The listing builds one solid part. Answer for the finished solid, in the listing's coordinates (mm). A direction names the side the tool comes from. Round coordinates to 2 decimals unless told otherwise and drop trailing zeros. Order: outer loops, then holes, each group sorted by start corner. A loop starts at its lowest first (then second) coordinate and runs counter-clockwise, first axis right, second up. Notation, with made-up numbers: (-4, -21) - (6, -21) arc R16 ccw to (6, 7) - close; hole circle Ø6 at (28, 39.25). An arc over 180 degrees is marked (long way). Write item = value, one per line.
from build123d import *

# Parameters (mm, degrees)
SKETCH1_R           = 2.25
SKETCH1_R_2         = 6.35
BOSS_EXTRUDE1_DEPTH = 12.7
FILLET1_R           = 6.35
FILLET3_R           = 6.35
FILLET5_R           = 2.5
FILLET4_R           = 1
CUT_EXTRUDE1_REACH  = 104.568
SKETCH2_R           = 2.25


with BuildPart() as part:
    # Sketch1 → Boss-Extrude1 (new body)
    # profile 1 of 2: a face of its own
    with BuildSketch(Plane(origin=(0, 0, 0), x_dir=(0, 0, -1), z_dir=(1, 0, 0))):
        with BuildLine():
            Line((-6.35, 76.319743879), (-6.35, 11.3))
            Line((-6.35, 11.3), (-31.75, 11.3))
            Line((-31.75, 11.3), (-31.75, 4.95))
            Line((-31.75, 4.95), (-6.35, 4.95))
            Line((-6.35, 4.95), (-6.35, -6.35))
            Line((-6.35, -6.35), (6.35, -6.35))
            Line((6.35, -6.35), (6.35, 11.3))
            Line((6.35, 11.3), (6.35, 81.580256121))
            Line((6.35, 81.580256121), (-11.859871939, 99.790128061))
            ThreePointArc((-11.859871939, 99.790128061), (-10.483364969, 97.730039796), (-10, 95.3))
            ThreePointArc((-10, 95.3), (-13.919960204, 89.433364969), (-20.840128061, 90.809871939))
            Line((-20.840128061, 90.809871939), (-6.35, 76.319743879))
        make_face()
        Circle(SKETCH1_R, mode=Mode.SUBTRACT)
    # profile 2 of 2: a face of its own
    with BuildSketch(Plane(origin=(0, 0, 0), x_dir=(0, 0, -1), z_dir=(1, 0, 0))):
        with Locations((-16.35, 95.3)):
            Circle(SKETCH1_R_2)
        with Locations((-16.35, 95.3)):
            Circle(SKETCH1_R, mode=Mode.SUBTRACT)
    extrude(amount=BOSS_EXTRUDE1_DEPTH)

    # Fillet1
    fillet1_edges = [part.edges().sort_by_distance(p)[0] for p in [
        (6.35, 81.580256121, -6.35),
        (6.35, 76.319743879, 6.35),
        (6.35, -6.35, -6.35),
        (6.35, -6.35, 6.35),
    ]]
    fillet(fillet1_edges, radius=FILLET1_R - 0.0001)  # a hair under: the kernel refuses the full size

    # Fillet3
    fillet3_edges = [part.edges().sort_by_distance(p)[0] for p in [
        (0, 8.125, 31.75),
        (12.7, 8.125, 31.75),
    ]]
    fillet(fillet3_edges, radius=FILLET3_R - 0.0001)  # a hair under: the kernel refuses the full size

    # Fillet5
    fillet5_edges = [part.edges().sort_by_distance(p)[0] for p in [
        (6.35, 4.95, 6.35),
    ]]
    fillet(fillet5_edges, radius=FILLET5_R)

    # Fillet4
    fillet4_edges = [part.edges().sort_by_distance(p)[0] for p in [
        (12.7, 99.790128061, 20.840128061),
        (0, 11.3, 15.87505),
        (0, 42.49476459, 6.35),
        (0, 99.790128061, 20.840128061),
        (0, 91.615113416, 3.684857295),
        (12.7, 42.49476459, 6.35),
        (6.35, 11.3, 6.35),
        (12.7, 11.3, 15.87505),
        (0, 39.474970711, -6.35),
        (0, 84.494729234, 14.524985355),
        (0, -4.49015735, 4.49015735),
        (0, -4.49015735, -4.49015735),
        (0, 81.380042949, -5.866642643),
        (12.7, 39.474970711, -6.35),
        (12.7, 84.494729234, 14.524985355),
        (12.7, -4.49015735, 4.49015735),
        (12.7, -4.49015735, -4.49015735),
        (12.7, 81.380042949, -5.866642643),
        (0, 76.119530706, 6.833357357),
        (12.7, 76.119530706, 6.833357357),
        (0, 4.95, 17.12505),
        (12.7, 4.95, 17.12505),
        (10.84015735, 4.95, 29.89015735),
        (1.85984265, 4.95, 29.89015735),
        (10.84015735, 11.3, 29.89015735),
        (1.85984265, 11.3, 29.89015735),
        (12.7, 91.615113416, 3.684857295),
        (0, 1.22495, 6.35),
        (12.7, 1.22495, 6.35),
        (0, 4.217766953, 7.082233047),
        (12.7, 4.217766953, 7.082233047),
    ]]
    fillet(fillet4_edges, radius=FILLET4_R)

    # Sketch2 → Cut-Extrude1 (cut, up to next)
    with BuildSketch(Plane.XZ.offset(-4.95), mode=Mode.PRIVATE) as cut_extrude1_sk1:
        with Locations(Location((6.35, 12.7, 0), (0, 0, 270))):
            Circle(SKETCH2_R)
    cut_extrude1_tool1 = extrude(cut_extrude1_sk1.sketch, amount=-CUT_EXTRUDE1_REACH, mode=Mode.PRIVATE) & part.part
    # Sketch2 → Cut-Extrude1 (cut, up to next)
    with BuildSketch(Plane.XZ.offset(-4.95), mode=Mode.PRIVATE) as cut_extrude1_sk2:
        with Locations(Location((6.35, 25.4, 0), (0, 0, 270))):
            Circle(SKETCH2_R)
    cut_extrude1_tool2 = extrude(cut_extrude1_sk2.sketch, amount=-CUT_EXTRUDE1_REACH, mode=Mode.PRIVATE) & part.part
    add(cut_extrude1_tool1.solids().sort_by_distance((6.35, 4.95, 12.7))[0], mode=Mode.SUBTRACT)
    add(cut_extrude1_tool2.solids().sort_by_distance((6.35, 4.95, 25.4))[0], mode=Mode.SUBTRACT)


solid = part.part
Q1. Section B-B on x = 2.5 is taken. Count the separate pieces of the cut face and the enclosed holes in it, then the cut area to 3 significant figures.
Model answer:
separate_pieces = 1
enclosed_holes = 2
area = 1,550 mm^2
Q2. Section A-A on y = 39 is taken. Determine the outline of the cut face in (x, z), then the cut area to 3 significant figures.
Model answer:
outline = (0, -5.35) arc R1 ccw to (1, -6.35) - (11.7, -6.35) arc R1 ccw to (12.7, -5.35) - (12.7, 5.35) arc R1 ccw to (11.7, 6.35) - (1, 6.35) arc R1 ccw to (0, 5.35) - close
area = 160 mm^2
Q3. Find the intervals of material crossed by line 1 (X direction, y = 8.5, z = 25.4); line 2 (Y direction, x = 5, z = 16); line 3 (Y direction, x = 4, z = 16.35), in increasing order. Write a range as from..to.
Model answer:
line_1 = 0..4.1, 8.6..12.7
line_2 = 4.95..11.3, 85.97..93.08, 97.52..101.64
line_3 = 4.95..11.3, 86.32..93.05, 97.55..101.65
Q4. For faces 5 (the face through (6.425, 76.152, 6.847)), 6 (the face through (6, 1, 6.35)), 7 (the face through (0.301, 84.785, 14.412)), determine the directions among +Z, -Z, +X, -X, +Y, -Y from which every point of the face is accessible in a straight line to the end or side of a thin tool.
Model answer:
face_5 = +Z, +X, -X
face_6 = +Z, +X, -X, -Y
face_7 = +Z, -X
Q5. Determine the mould class of faces 1 (the face through (5.49, 8.08, 10.62)), 2 (the face through (12.7, 52, 3)), 3 (the face through (1.81, 8.09, 29.84)), 4 (the face through (6.449, 8.081, 27.648)) for opening direction X: released by +X, released by -X, zero draft, split by the parting line, or undercut.
Model answer:
face_1 = undercut
face_2 = released by +X
face_3 = released by -X
face_4 = undercut
Q6. Flat-ended cylindrical pins translate along their axes: P1, Ø2, axis at x = 5.5, y = 1.5, coming from the +Z side; P2, Ø3, axis at x = 9, y = 31, coming from the +Z side; P3, Ø5, axis at x = 6.35, z = 12.7, coming from the -Y side; P4, Ø4, axis at y = 95.3, z = 16.35, coming from the +X side. Find the tip coordinate at first contact, or state that the pin passes through.
Model answer:
P1 = 6.35
P2 = 6.35
P3 = 4.95
P4 = through
